```python
from build123d import *

# Parameters (mm, degrees)
BOSS_EXTRUDE1_DEPTH            = 57
SKETCH3_R                      = 4
CUT_EXTRUDE1_DEPTH             = 94.743374336
CBORE_FOR_M8_SHCS2_D           = 9
CBORE_FOR_M8_SHCS2_CBORE_D     = 13.5
CBORE_FOR_M8_SHCS2_CBORE_DEPTH = 20
SKETCH7_W                      = 30
SKETCH7_H                      = 57
BOSS_EXTRUDE2_DEPTH            = 10
BOSS_EXTRUDE3_DEPTH            = 5
BOSS_EXTRUDE3_DEPTH_BACK       = 5
SKETCH9_W                      = 25
SKETCH9_H                      = 57
BOSS_EXTRUDE4_DEPTH            = 10
BOSS_EXTRUDE5_DEPTH            = 5
BOSS_EXTRUDE5_DEPTH_BACK       = 5
CUT_EXTRUDE2_DEPTH             = 10
FILLET1_R                      = 7
CHAMFER1_SIZE                  = 12
M8_CLEARANCE_HOLE1_D           = 9


with BuildPart() as part:
    # Sketch2 → Boss-Extrude1 (new body)
    with BuildSketch(Plane.XY):
        Polygon((0, 0), (54.389155461, 45.637920288), (54.389155461, -50.8), (0, -50.8), align=None)
    extrude(amount=BOSS_EXTRUDE1_DEPTH)

    # Sketch3 → Cut-Extrude1 (cut, through all)
    with BuildSketch(Plane(origin=(0, 0, 0), x_dir=(0.7660444431189817, 0.6427876096865353, 0), z_dir=(-0.6427876096865353, 0.7660444431189817, 0))):
        with Locations(Location((38.5, -7.5, 0), (0, 0, 180))):
            Circle(SKETCH3_R)
        with Locations(Location((38.5, -49.5, 0), (0, 0, 180))):
            Circle(SKETCH3_R)
    extrude(amount=-CUT_EXTRUDE1_DEPTH, mode=Mode.SUBTRACT)

    # CBORE for M8 SHCS2 (through all)
    with Locations(Plane(origin=(32.139380484, -38.302222156, 0), x_dir=(0.7660444431189817, 0.6427876096865353, 0), z_dir=(0.6427876096865353, -0.7660444431189817, 0))):
        with Locations((38.5, 49.5), (38.5, 7.5)):
            CounterBoreHole(CBORE_FOR_M8_SHCS2_D / 2, CBORE_FOR_M8_SHCS2_CBORE_D / 2, CBORE_FOR_M8_SHCS2_CBORE_DEPTH)

    # Sketch7 → Boss-Extrude2 (add)
    with BuildSketch(Plane.XZ.offset(50.8)):
        with Locations((69.389155461, 28.5)):
            Rectangle(SKETCH7_W, SKETCH7_H)
    extrude(amount=-BOSS_EXTRUDE2_DEPTH)

    # Sketch8 → Boss-Extrude3 (add, two sides: drawn at the far end of the back side and taken through both)
    with BuildSketch(Plane.XY.offset(28.5).offset(-BOSS_EXTRUDE3_DEPTH_BACK)):
        Polygon((84.389155461, -40.8), (54.389155461, -0.8), (54.389155461, -40.8), align=None)
    extrude(amount=BOSS_EXTRUDE3_DEPTH + BOSS_EXTRUDE3_DEPTH_BACK)

    # Sketch9 → Boss-Extrude4 (add)
    with BuildSketch(Plane.XZ.offset(50.8)):
        with Locations((-12.5, 28.5)):
            Rectangle(SKETCH9_W, SKETCH9_H)
    extrude(amount=-BOSS_EXTRUDE4_DEPTH)

    # Sketch10 → Boss-Extrude5 (add, two sides: drawn at the far end of the back side and taken through both)
    with BuildSketch(Plane.XY.offset(28.5).offset(-BOSS_EXTRUDE5_DEPTH_BACK)):
        Polygon((-25, -40.8), (0, -15.8), (0, -40.8), align=None)
    extrude(amount=BOSS_EXTRUDE5_DEPTH + BOSS_EXTRUDE5_DEPTH_BACK)

    # Sketch11 → Cut-Extrude2 (cut)
    with BuildSketch(Plane(origin=(0, 0, 0), x_dir=(-1, 0, 0), z_dir=(0, 0, -1))):
        with BuildLine():
            Line((-38.389155461, -7.8), (-16, -7.8))
            ThreePointArc((-16, -7.8), (-10.343145751, -10.143145751), (-8, -15.8))
            Line((-8, -15.8), (-8, -34.8))
            ThreePointArc((-8, -34.8), (-10.343145751, -40.456854249), (-16, -42.8))
            Line((-16, -42.8), (-38.389155461, -42.8))
            ThreePointArc((-38.389155461, -42.8), (-44.046009711, -40.456854249), (-46.389155461, -34.8))
            Line((-46.389155461, -34.8), (-46.389155461, -15.8))
            ThreePointArc((-46.389155461, -15.8), (-44.046009711, -10.143145751), (-38.389155461, -7.8))
        make_face()
    cut_extrude2 = extrude(amount=-CUT_EXTRUDE2_DEPTH, mode=Mode.SUBTRACT)

    # Mirror1: Cut-Extrude2 across plane
    add(cut_extrude2.mirror(Plane.XY.offset(28.5)), mode=Mode.SUBTRACT)

    # Fillet1
    fillet1_edges = [part.edges().sort_by_distance(p)[0] for p in [
        (54.389155461, -40.8, 45.25),
        (54.389155461, -40.8, 11.75),
        (0, -40.8, 11.75),
        (0, -40.8, 45.25),
    ]]
    fillet(fillet1_edges, radius=FILLET1_R)

    # Chamfer1
    chamfer1_edges = [part.edges().sort_by_distance(p)[0] for p in [
        (84.389155461, -45.8, 57),
        (84.389155461, -45.8, 0),
    ]]
    chamfer(chamfer1_edges, length=CHAMFER1_SIZE)

    # M8 Clearance Hole1 (through all)
    with Locations(Plane(origin=(0, -40.8, 0), x_dir=(1, 0, 0), z_dir=(0, 1, 0))):
        with Locations((72.389155461, -43), (72.389155461, -14), (-15, -10), (-15, -47)):
            Hole(M8_CLEARANCE_HOLE1_D / 2)


solid = part.part
```
The model under review builds one solid part; all positions refer to its coordinate system, in mm. A direction names the side the tool comes from. Give positions to 0.01 mm unless a question says otherwise; leave off trailing zeros. Write each loop counter-clockwise with the first axis right and the second up, starting at its lowest first coordinate (ties: lowest second). Pieces come first, ordered by that corner, then holes. Notation, with made-up numbers: M 45,-36.5 L 56,-36.5 A21 cw 56,-7.5 Z; hole C 87,37 d3. An arc over 180 degrees is marked long. Write item = value, one per line. Start each with the question number.
Q1. Clearance check with flat-ended pins moving along their axes: pin 1 (17 mm diameter, centred on y = 12.5, z = 30.5, fed in from +X); pin 2 (3 mm diameter, centred on y = -29, z = 52.5, fed in from -X); pin 3 (12 mm diameter, centred on y = 7.5, z = 17.5, fed in from -X). State where each tip first meets the part, or that it passes through.
Q2. Mouldability with a two-part tool opening along X and no side actions: class faces 4 (the face through (84.389, -46, 28)), 5 (the face through (-2.1, -38.8, 45.4)), 6 (the face through (-11.4, -45.9, 12.7)) as released by +X, released by -X, zero draft, split by the parting line, or undercut.
Q3. For line 1 (Y direction, x = 65, z = 3.5); line 2 (X direction, y = -48.25, z = 43); line 3 (Z direction, x = -0.5, y = -24), list the stretches that pass through material, from the lowest coordinate up.
Q4. We need section A-A (x = -15). State the section outline as (y, z) points.
Q5. We need section B-B (z = 16). State the section outline as (x, y) points, plus the area to 3 significant figures.
Q6. Machinability: for faces 1 (the face through (46.389, -25, 5)), 2 (the face through (47.555, 0.741, 3.094)), 3 (the face through (0, -13, 28)), which of the approach directions +Z, -Z, +X, -X, +Y, -Y give a long, thin tool a straight path to every point of the face, cutting with its end or side? Answer none if there is none.
Q7. We need section C-C (y = -17.5). State the section outline as (x, z) points.
Q8. We need section D-D (y = 35.5). State the section outline as (x, z) points, plus the area to 3 significant figures.
Result set:
q1.pin_1 = 54.39
q1.pin_2 = 0
q1.pin_3 = 1.79
q2.face_4 = released by +X
q2.face_5 = released by -X
q2.face_6 = undercut
q3.line_1 = -50.8 to -40.8
q3.line_2 = -25 to -17.06, -12.94 to 67.89, 76.89 to 84.39
q3.line_3 = 23.5 to 33.5
q4.outline = M -50.8,0 L -40.8,0 L -40.8,5.5 L -50.8,5.5 Z; M -50.8,14.5 L -40.8,14.5 L -40.8,23.5 L -30.8,23.5 L -30.8,33.5 L -40.8,33.5 L -40.8,42.5 L -50.8,42.5 Z; M -50.8,51.5 L -40.8,51.5 L -40.8,57 L -50.8,57 Z
q5.outline = M -25,-50.8 L 68.36,-50.8 L 68.36,-40.8 L 61.39,-40.8 A7 cw 54.39,-33.8 L 54.39,45.64 L 0,0 L 0,-33.8 A7 cw -7,-40.8 L -25,-40.8 Z; M 76.42,-50.8 L 84.39,-50.8 L 84.39,-40.8 L 76.42,-40.8 Z
q5.area = 4,490 mm2
q6.face_1 = -Z
q6.face_2 = none
q6.face_3 = -X, +Y
q7.outline = M -1.7,23.5 L 0,23.5 L 0,0 L 8,0 L 8,10 L 46.39,10 L 46.39,0 L 54.39,0 L 54.39,23.5 L 66.91,23.5 L 66.91,33.5 L 54.39,33.5 L 54.39,57 L 46.39,57 L 46.39,47 L 8,47 L 8,57 L 0,57 L 0,33.5 L -1.7,33.5 Z
q8.outline = M 42.31,0 L 54.39,0 L 54.39,57 L 42.31,57 Z
q8.area = 689 mm2
